Check sheet for the modelled part. Datum: model origin and axes. Units: mm. Face numbers are marked on the shaded views. A direction names the side the tool comes from. Give positions to 0.01 mm unless a question says otherwise; leave off trailing zeros. Write each loop counter-clockwise with the first axis right and the second up, starting at its lowest first coordinate (ties: lowest second). Pieces come first, ordered by that corner, then holes. Notation, with made-up numbers: M -25.5,-13 L -1.5,-13 A17 ccw -1.5,10 Z; hole C 70,43.5 d6. An arc over 180 degrees is marked long. One line per item, written item: value. Start each with the question number.
from build123d import *

# Parameters (mm, degrees)
BOSS_EXTRU_1_DEPTH      = 25
ENL_V_MAT_EXTRU_1_DEPTH = 20
ENL_V_MAT_EXTRU_2_DEPTH = 45.21248121115924
ENL_V_MAT_EXTRU_4_DEPTH = 20
ENL_V_MAT_EXTRU_3_DEPTH = 45.21248121115924
CHANFREIN1_SIZE         = 1.2
BOSS_EXTRU_2_START      = 3
BOSS_EXTRU_2_DEPTH      = 3
ENL_V_MAT_EXTRU_5_REACH = 47.001
ESQUISSE7_W             = 1.399999999999995
ESQUISSE7_H             = 20
CHANFREIN2_SIZE2        = 4
CHANFREIN2_SIZE         = 2.309401077
ENL_V_MAT_EXTRU_6_REACH = 60.237
CHANFREIN3_SIZE2        = 4
CHANFREIN3_SIZE         = 2.309401077


with BuildPart() as part:
    # Esquisse1 → Boss.-Extru.1 (new body)
    with BuildSketch(Plane.XY):
        with BuildLine():
            Line((-22.99038105676658, 1.7264973081037391), (-12.990381056766578, 19.047005383792516))
            ThreePointArc((-12.990381056766578, 19.047005383792516), (9.5e-16, 26.547005383792516), (12.990381056766578, 19.047005383792513))
            Line((12.990381056766578, 19.047005383792513), (22.990381056766577, 1.726497308103746))
            ThreePointArc((22.990381056766577, 1.726497308103746), (22.99038105676658, -13.273502691896258), (9.999999999999996, -20.77350269189626))
            Line((9.999999999999996, -20.77350269189626), (-10, -20.773502691896258))
            ThreePointArc((-10, -20.773502691896258), (-22.99038105676658, -13.273502691896255), (-22.99038105676658, 1.7264973081037391))
        make_face()
        with BuildLine():
            Line((-18.66025403784439, -0.7735026918962613), (-8.66025403784439, 16.547005383792516))
            ThreePointArc((-8.66025403784439, 16.547005383792516), (-2.69e-15, 21.547005383792516), (8.660254037844384, 16.547005383792516))
            Line((8.660254037844384, 16.547005383792516), (18.660254037844386, -0.7735026918962474))
            ThreePointArc((18.660254037844386, -0.7735026918962474), (18.660254037844393, -10.773502691896258), (10, -15.773502691896258))
            Line((10, -15.773502691896258), (-10, -15.773502691896258))
            ThreePointArc((-10, -15.773502691896258), (-18.66025403784439, -10.773502691896262), (-18.66025403784439, -0.7735026918962613))
        make_face(mode=Mode.SUBTRACT)
    extrude(amount=BOSS_EXTRU_1_DEPTH)

    # Esquisse2 → Enlèv. mat.-Extru.1 (cut)
    with BuildSketch(Plane.XY.offset(25)):
        Polygon((-10.914359353944898, 12.642780450695335), (-12.300000000000002, 13.442780450695334), (-11.600000000000003, 14.655216015993549), (-10.2143593539449, 13.855216015993548), align=None)
        Polygon((10.214359353944896, 13.855216015993548), (11.6, 14.655216015993549), (12.299999999999999, 13.442780450695334), (10.914359353944896, 12.642780450695334), align=None)
    extrude(amount=-ENL_V_MAT_EXTRU_1_DEPTH, mode=Mode.SUBTRACT)

    # Esquisse3 → Enlèv. mat.-Extru.2 (cut, through all)
    with BuildSketch(Plane.XY.offset(25)):
        Polygon((-10.064359353944898, 14.115023637128878), (-11.709807621135333, 15.06502363712888), (-12.709807621135335, 13.332972829560003), (-11.064359353944898, 12.382972829560003), align=None)
    enl_v_mat_extru_2 = extrude(amount=-ENL_V_MAT_EXTRU_2_DEPTH, mode=Mode.SUBTRACT)

    # Symétrie1: Enlèv. mat.-Extru.2 across plane
    add(enl_v_mat_extru_2.mirror(Plane(origin=(0, 0, 0), x_dir=(0, 0, 1), z_dir=(1, 0, 0))), mode=Mode.SUBTRACT)

    # Esquisse6 → Enlèv. mat.-Extru.4 (cut)
    with BuildSketch(Plane(origin=(0, 0, 0), x_dir=(-1, 0, 0), z_dir=(0, 0, -1))):
        Polygon((11.250000000000002, 12.061433798642659), (15.147114317029969, 14.31143379864266), (18.297114317029976, 8.855473754800698), (14.4, 6.605473754800695), align=None)
        Polygon((-11.249999999999998, 12.061433798642659), (-15.14711431702997, 14.311433798642657), (-18.297114317029973, 8.855473754800693), (-14.399999999999997, 6.605473754800696), align=None)
    extrude(amount=-ENL_V_MAT_EXTRU_4_DEPTH, mode=Mode.SUBTRACT)

    # Esquisse5 → Enlèv. mat.-Extru.3 (cut, through all)
    with BuildSketch(Plane.XY.offset(25)):
        with BuildLine():
            Line((-9.093266739736611, 16.797005383792516), (-10.497372055837118, 14.365023637128878))
            Line((-10.497372055837118, 14.365023637128878), (-11.497372055837118, 12.632972829560003))
            Line((-11.497372055837118, 12.632972829560003), (-19.093266739736613, -0.5235026918962613))
            ThreePointArc((-19.093266739736613, -0.5235026918962613), (-19.09326673973661, -11.023502691896262), (-10.000000000000002, -16.273502691896258))
            Line((-10.000000000000002, -16.273502691896258), (10.000000000000004, -16.273502691896258))
            ThreePointArc((10.000000000000004, -16.273502691896258), (19.09326673973661, -11.023502691896251), (19.093266739736602, -0.523502691896249))
            Line((19.093266739736602, -0.523502691896249), (11.497372055837113, 12.632972829560005))
            Line((11.497372055837113, 12.632972829560005), (10.497372055837118, 14.36502363712888))
            Line((10.497372055837118, 14.36502363712888), (9.0932667397366, 16.797005383792516))
            ThreePointArc((9.0932667397366, 16.797005383792516), (-2.66e-15, 22.047005383792516), (-9.093266739736611, 16.797005383792516))
        make_face()
        with BuildLine():
            Line((-8.66025403784439, 16.547005383792516), (-10.064359353944898, 14.115023637128878))
            Line((-10.064359353944898, 14.115023637128878), (-11.064359353944894, 12.382972829560005))
            Line((-11.064359353944894, 12.382972829560005), (-18.66025403784439, -0.7735026918962613))
            ThreePointArc((-18.66025403784439, -0.7735026918962613), (-18.66025403784439, -10.773502691896262), (-10, -15.773502691896258))
            Line((-10, -15.773502691896258), (10.000000000000002, -15.77350269189626))
            ThreePointArc((10.000000000000002, -15.77350269189626), (18.66025403784439, -10.773502691896255), (18.660254037844386, -0.7735026918962474))
            Line((18.660254037844386, -0.7735026918962474), (11.064359353944898, 12.382972829560003))
            Line((11.064359353944898, 12.382972829560003), (10.064359353944898, 14.115023637128878))
            Line((10.064359353944898, 14.115023637128878), (8.660254037844384, 16.547005383792516))
            ThreePointArc((8.660254037844384, 16.547005383792516), (-2.69e-15, 21.547005383792516), (-8.66025403784439, 16.547005383792516))
        make_face(mode=Mode.SUBTRACT)
    extrude(amount=-ENL_V_MAT_EXTRU_3_DEPTH, mode=Mode.SUBTRACT)

    # Chanfrein1
    chanfrein1_edges = [part.edges().sort_by_distance(p)[0] for p in [
        (22.99038105676658, -13.27350269189626, 25),
        (11.103589838486222, 14.715023637128876, 25),
        (-11.103589838486226, 14.71502363712888, 25),
        (-9.795319397786868, 15.581014510460694, 25),
        (9.795319397786855, 15.581014510460696, 25),
        (-7.11e-15, 22.047005383792516, 25),
        (-15.295319397786866, 6.054735068831872, 25),
        (-19.09326673973661, -11.023502691896262, 25),
        (1.78e-15, -16.273502691896258, 25),
        (19.093266739736606, -11.023502691896253, 25),
        (15.295319397786855, 6.054735068831873, 25),
        (17.990381056766577, 10.386751345948129, 25),
        (2.66e-15, 26.547005383792516, 25),
        (-17.99038105676658, 10.386751345948127, 25),
        (-22.99038105676658, -13.273502691896258, 25),
        (-12.209807621135333, 14.19899823334444, 25),
        (-12.103589838486226, 12.982972829560003, 25),
        (-1.78e-15, -20.77350269189626, 25),
        (12.209807621135335, 14.19899823334444, 25),
        (12.103589838486222, 12.982972829560001, 25),
    ]]
    chamfer(chanfrein1_edges, length=CHANFREIN1_SIZE)

    # Esquisse4 → Boss.-Extru.2 (add)
    with BuildSketch(Plane(origin=(0, 0, 0), x_dir=(-1, 0, 0), z_dir=(0, 0, -1)).offset(BOSS_EXTRU_2_START)):
        with BuildLine():
            Line((22.99038105676658, 1.7264973081037323), (12.990381056766578, 19.047005383792516))
            ThreePointArc((12.990381056766578, 19.047005383792516), (8.9e-16, 26.547005383792513), (-12.990381056766573, 19.047005383792513))
            Line((-12.990381056766573, 19.047005383792513), (-22.990381056766577, 1.726497308103746))
            ThreePointArc((-22.990381056766577, 1.726497308103746), (-22.99038105676658, -13.273502691896255), (-10.000000000000004, -20.773502691896258))
            Line((-10.000000000000004, -20.773502691896258), (9.999999999999996, -20.773502691896258))
            ThreePointArc((9.999999999999996, -20.773502691896258), (22.990381056766577, -13.273502691896262), (22.99038105676658, 1.7264973081037323))
        make_face()
    extrude(amount=-BOSS_EXTRU_2_DEPTH)

    # Esquisse7 → Enlèv. mat.-Extru.5 (cut, up to next)
    with BuildSketch(Plane(origin=(-2.5958946838994956, 4.496221483611885, 0), x_dir=(0.866025403784439, 0.4999999999999994, 0), z_dir=(-0.4999999999999994, 0.866025403784439, 0)), mode=Mode.PRIVATE) as enl_v_mat_extru_5_sk1:
        with Locations((16.973502691896265, -10)):
            Rectangle(ESQUISSE7_W, ESQUISSE7_H)
    enl_v_mat_extru_5_tool1 = extrude(enl_v_mat_extru_5_sk1.sketch, amount=-ENL_V_MAT_EXTRU_5_REACH, mode=Mode.PRIVATE) & part.part
    enl_v_mat_extru_5 = enl_v_mat_extru_5_tool1.solids().sort_by_distance((12.10359, 12.982973, 10))[0]
    add(enl_v_mat_extru_5, mode=Mode.SUBTRACT)

    # Symétrie2: Enlèv. mat.-Extru.5 across plane
    add(enl_v_mat_extru_5.mirror(Plane(origin=(0, 0, 0), x_dir=(0, 0, 1), z_dir=(1, 0, 0))), mode=Mode.SUBTRACT)

    # Chanfrein2
    chanfrein2_edges = [part.edges().sort_by_distance(p)[0] for p in [
        (13.16519237886467, 9.74422329218035, 20),
    ]]
    chanfrein2_side = [part.faces().sort_by_distance(p)[0] for p in [
        (13.16519237886467, 9.74422329218035, 20.04618802153517),
    ]]
    chamfer(chanfrein2_edges, length=CHANFREIN2_SIZE - 0.0001, length2=CHANFREIN2_SIZE2 - 0.0001, reference=chanfrein2_side[0])  # a hair under: the kernel refuses the full size

    # Esquisse8 → Enlèv. mat.-Extru.6 (cut, up to next)
    with BuildSketch(Plane(origin=(17.557368354874363, 10.13675134594814, 0), x_dir=(0, 0, 1), z_dir=(-0.8660254037844385, -0.5000000000000004, 0)), mode=Mode.PRIVATE) as enl_v_mat_extru_6_sk1:
        Polygon((3.0000000000000004, 4.320508075688777), (5.3e-16, 4.320508075688777), (8.7e-16, -0.9794919243112247), (3.000000000000001, -0.9794919243112244), align=None)
    enl_v_mat_extru_6_tool1 = extrude(enl_v_mat_extru_6_sk1.sketch, amount=-ENL_V_MAT_EXTRU_6_REACH, mode=Mode.PRIVATE) & part.part
    enl_v_mat_extru_6 = enl_v_mat_extru_6_tool1.solids().sort_by_distance((16.722114, 11.583454, 1.5))[0]
    add(enl_v_mat_extru_6, mode=Mode.SUBTRACT)

    # Symétrie3: Enlèv. mat.-Extru.6 across plane
    add(enl_v_mat_extru_6.mirror(Plane(origin=(0, 0, 0), x_dir=(0, 0, 1), z_dir=(1, 0, 0))), mode=Mode.SUBTRACT)

    # Chanfrein3
    chanfrein3_edges = [part.edges().sort_by_distance(p)[0] for p in [
        (-13.16519237886467, 9.74422329218035, 20),
    ]]
    chanfrein3_side = [part.faces().sort_by_distance(p)[0] for p in [
        (-13.16519237886467, 9.74422329218035, 20.04618802153517),
    ]]
    chamfer(chanfrein3_edges, length=CHANFREIN3_SIZE - 0.0001, length2=CHANFREIN3_SIZE2 - 0.0001, reference=chanfrein3_side[0])  # a hair under: the kernel refuses the full size


solid = part.part
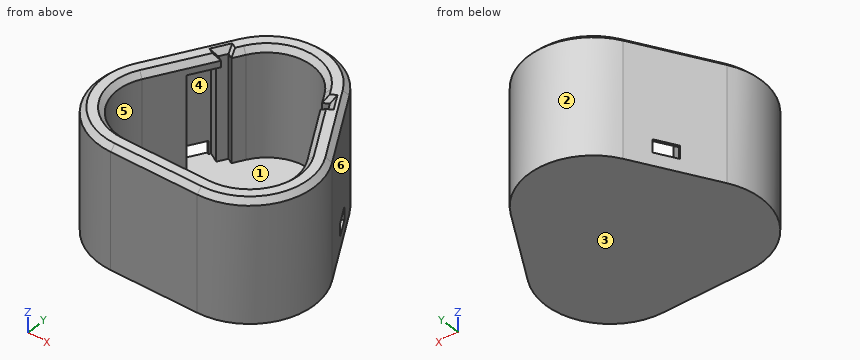
1) Gauge pin test, flat ends, axial feed: pin 1 (2 mm diameter, centred on x = -13.5, z = 1.5, fed in from -Y); pin 2 (6 mm diameter, centred on x = 0.5, y = 20.5, fed in from +Z); pin 3 (6 mm diameter, centred on x = 13, z = 15, fed in from +Y); pin 4 (3 mm diameter, centred on y = 10.5, z = 14, fed in from -X). Record the tip position at first contact, or that the pin passes through.
2) Cross-section at A-A (z = 23). Record the boundary of the cut face in (x, y), plus the area to 3 significant figures.
3) Material ranges on L1, parallel to Y at x = 15, z = 18; L2, parallel to Z at x = 4, y = -12.5; L3, parallel to X at y = -3, z = 7, recorded low to high. Write a range as from..to.
4) Cross-section at B-B (z = 11.25). Record the boundary of the cut face in (x, y).
5) Tool access check on the marked faces 4, 5 and 6. Record the directions out of +Z, -Z, +X, -X, +Y, -Y that give a thin tool (end or side, any length) a straight path to the whole face; none if there is none.
6) Draft check along X on the marked faces 1, 2 and 3. Enter one of: released by +X, released by -X, zero draft, split by the parting line, or undercut.
Data:
1. pin 1: stops at y = -20.56
1. pin 2: stops at z = 25
1. pin 3: stops at y = 22.73
1. pin 4: stops at x = -18.79
2. outline: M -22.99,1.73 A15 ccw -10,-20.77 L 10,-20.77 A15 ccw 22.99,1.73 L 12.99,19.05 A15 ccw -12.99,19.05 Z; hole M -19.09,-0.52 A10.5 ccw -10,-16.27 L 10,-16.27 A10.5 ccw 19.09,-0.52 L 11.5,12.63 L 12.71,13.33 L 11.71,15.07 L 10.5,14.37 L 9.09,16.8 A10.5 ccw -9.09,16.8 L -10.5,14.37 L -11.71,15.07 L -12.71,13.33 L -11.5,12.63 Z
2. area: 625 mm2
3. L1: y = -19.92..-15.01, 6.57..6.95, 14.23..15.57
3. L2: z = -3..0
3. L3: x = -24.74..-20.13, 20.13..24.74
4. outline: M -22.99,1.73 A15 ccw -10,-20.77 L 10,-20.77 A15 ccw 22.99,1.73 L 12.99,19.05 A15 ccw -12.99,19.05 Z; hole M -19.09,-0.52 A10.5 ccw -10,-16.27 L 10,-16.27 A10.5 ccw 19.09,-0.52 L 14.83,6.86 L 18.3,8.86 L 15.15,14.31 L 12.9,13.01 L 11.71,15.07 L 10.5,14.37 L 9.09,16.8 A10.5 ccw -9.09,16.8 L -10.5,14.37 L -11.71,15.07 L -12.9,13.01 L -15.15,14.31 L -18.3,8.86 L -14.83,6.86 Z
5. face 4: none
5. face 5: +Z
5. face 6: +Z, -Z, +X, +Y
6. face 1: undercut
6. face 2: split by the parting line
6. face 3: zero draft
